```python
from build123d import *

# Parameters (mm, degrees)
SKETCH2_R           = 19
SKETCH2_R_2         = 10
SKETCH2_R_3         = 3
BOSS_EXTRUDE1_DEPTH = 33
SKETCH2_3_R         = 10
SKETCH2_3_R_2       = 3
BOSS_EXTRUDE2_DEPTH = 5
SKETCH2_4_R         = 3
BOSS_EXTRUDE3_DEPTH = 17.5
SKETCH4_R           = 5
BOSS_EXTRUDE4_DEPTH = 25
SKETCH5_R           = 1.575
CUT_EXTRUDE1_DEPTH  = 6


with BuildPart() as part:
    # Sketch2 → Boss-Extrude1 (new body)
    # profile 1 of 3: a face of its own
    with BuildSketch(Plane.XY):
        Circle(SKETCH2_R)
        Circle(SKETCH2_R_2, mode=Mode.SUBTRACT)
    # profile 2 of 3: a face of its own
    with BuildSketch(Plane.XY):
        Circle(SKETCH2_R_2)
        Circle(SKETCH2_R_3, mode=Mode.SUBTRACT)
    # profile 3 of 3: a face of its own
    with BuildSketch(Plane.XY):
        Circle(SKETCH2_R_3)
    extrude(amount=-BOSS_EXTRUDE1_DEPTH)

    # Sketch2_3 → Boss-Extrude2 (add)
    with BuildSketch(Plane.XY):
        Circle(SKETCH2_3_R)
        Circle(SKETCH2_3_R_2, mode=Mode.SUBTRACT)
    extrude(amount=BOSS_EXTRUDE2_DEPTH)

    # Sketch2_4 → Boss-Extrude3 (add)
    with BuildSketch(Plane.XY):
        Circle(SKETCH2_4_R)
    extrude(amount=BOSS_EXTRUDE3_DEPTH)

    # Sketch4 → Boss-Extrude4 (add)
    with BuildSketch(Plane(origin=(0, 0, 0), x_dir=(1, 0, 0), z_dir=(0, 1, 0))):
        with Locations(Location((0, 25.688557627, 0), (0, 0, 270))):
            Circle(SKETCH4_R)
    extrude(amount=-BOSS_EXTRUDE4_DEPTH)

    # Sketch5 → Cut-Extrude1 (cut)
    with BuildSketch(Plane.XY):
        with Locations((0, 15)):
            Circle(SKETCH5_R)
        with Locations((12.990381057, -7.5)):
            Circle(SKETCH5_R)
        with Locations((-12.990381057, -7.5)):
            Circle(SKETCH5_R)
        with Locations((8.030070109, 11.46812862)):
            Circle(SKETCH5_R)
        with Locations((5.916655664, -12.688309019)):
            Circle(SKETCH5_R)
        with Locations((-13.946725773, 1.220180398)):
            Circle(SKETCH5_R)
    extrude(amount=-CUT_EXTRUDE1_DEPTH, mode=Mode.SUBTRACT)


solid = part.part
```
Work out the finished part from the listing and answer in its coordinate system (mm). A direction names the side the tool comes from. Coordinates: 2 decimals unless noted, no trailing zeros. Write each loop counter-clockwise with the first axis right and the second up, starting at its lowest first coordinate (ties: lowest second). Pieces come first, ordered by that corner, then holes.
Q1. A cutting plane is placed at B-B, the plane y = -4. Give the vertices of the cut face in (x, z).
Q2. A cutting plane is placed at C-C, the plane z = 3.5. Give the vertices of the cut face in (x, y).
Q3. Find the intervals of material crossed by line 1 (Z direction, x = -4, y = 9); line 2 (Y direction, x = 0.5, z = -24); line 3 (Z direction, x = 15.5, y = -5.5), in increasing order.
Q4. Determine the mould class of faces 1 (the face through (2.1, 2.4, 5)), 2 (the face through (10.214, 16.021, -16.269)), 3 (the face through (13.837, -6.172, -2.958)) for opening direction Y: released by +Y, released by -Y, zero draft, split by the parting line, or undercut.
Q5. Each of these flat-tipped pins is pushed along its axis until it touches: pin 1 Ø8 at (x, z) = (1.5, -0.5) entering from +Y; pin 2 Ø8 at (x, z) = (11.5, -19) entering from -Y; pin 3 Ø1.9 at (x, y) = (12.99, -7.5) entering from +Z. Where does it stop, or does it pass through?
Q6. Which of the six approach directions +Z, -Z, +X, -X, +Y, -Y give full straight-line access (tool end or side, diameter ignored) to faces 4 (the face through (6, -13, -6)), 5 (the face through (1.5, -21.62, -20.92)), 6 (the face through (0, 0, -33))?
Q7. A cutting plane is placed at A-A, the plane x = 0. Give the vertices of the cut face in (y, z) (3 decimals), then the cut area to 3 significant figures.
Q8. A cutting plane is placed at D-D, the plane z = -4. Give the vertices of the cut face in (x, y) (3 decimals).
Findings below:
1. outline: (-18.57, -33) - (18.57, -33) - (18.57, 0) - (9.17, 0) - (9.17, 5) - (-9.17, 5) - (-9.17, 0) - (-18.57, 0) - close
2. outline: circle Ø20 at (0, 0)
3. line 1: z = -33 to 5
3. line 2: y = -25 to 18.99
3. line 3: z = -33 to 0
4. face 1: zero draft
4. face 2: split by the parting line
4. face 3: undercut
5. pin 1: stops at y = 19
5. pin 2: stops at y = -17.46
5. pin 3: stops at z = -6
6. face 4: +Z
6. face 5: -Y
6. face 6: -Z, +X, -X, +Y, -Y
7. outline: (-25, -30.689) - (-19, -30.689) - (-19, -33) - (19, -33) - (19, 0) - (16.575, 0) - (16.575, -6) - (13.425, -6) - (13.425, 0) - (10, 0) - (10, 5) - (3, 5) - (3, 17.5) - (-3, 17.5) - (-3, 5) - (-10, 5) - (-10, 0) - (-19, 0) - (-19, -20.689) - (-25, -20.689) - close
7. area: 1,470 mm2
8. outline: circle Ø38 at (0, 0); hole circle Ø3.15 at (-13.947, 1.22); hole circle Ø3.15 at (-12.99, -7.5); hole circle Ø3.15 at (0, 15); hole circle Ø3.15 at (5.917, -12.688); hole circle Ø3.15 at (8.03, 11.468); hole circle Ø3.15 at (12.99, -7.5)
